```python
from build123d import *

# Parameters (mm, degrees)
SKETCH_1_R                = 2.15
EXTRUDE_1_DEPTH           = 4
SKETCH_2_R                = 16.75
SKETCH_2_R_2              = 1.65
CUT_EXTRUDE_1_DEPTH       = 10
CUT_EXTRUDE_2_DEPTH       = 10
FILLET_1_R                = 1.5
HOLE_WIZARD_1_D           = 3.4
HOLE_WIZARD_1_CSINK_D     = 6.6
HOLE_WIZARD_1_CSINK_ANGLE = 90


with BuildPart() as part:
    # 草图1 → 凸台-拉伸1 (new body)
    with BuildSketch(Plane.XY):
        with BuildLine():
            Line((-52, 30), (-52, 8.75))
            Line((-52, 8.75), (-52, -8.75))
            Line((-52, -8.75), (-52, -30))
            Line((-52, -30), (-47.54, -30))
            ThreePointArc((-47.54, -30), (-44.004466094, -31.464466094), (-42.54, -35))
            Line((-42.54, -35), (-42.54, -37.5))
            ThreePointArc((-42.54, -37.5), (-38.982425028, -42.287422066), (-33.372235985, -40.262198963))
            ThreePointArc((-33.372235985, -40.262198963), (-30.171244586, -38.118753147), (-26.396349665, -38.887436588))
            ThreePointArc((-26.396349665, -38.887436588), (0, -47), (26.396349665, -38.887436588))
            ThreePointArc((26.396349665, -38.887436588), (30.171244586, -38.118753147), (33.372235985, -40.262198963))
            ThreePointArc((33.372235985, -40.262198963), (38.674773042, -42.369526686), (42.499484755, -38.135225128))
            Line((42.499484755, -38.135225128), (46.619156699, -5.971116201))
            ThreePointArc((46.619156699, -5.971116201), (47, 0), (46.619156699, 5.971116201))
            Line((46.619156699, 5.971116201), (42.499484755, 38.135225128))
            ThreePointArc((42.499484755, 38.135225128), (38.674773042, 42.369526686), (33.372235985, 40.262198963))
            ThreePointArc((33.372235985, 40.262198963), (30.171244586, 38.118753147), (26.396349665, 38.887436588))
            ThreePointArc((26.396349665, 38.887436588), (0, 47), (-26.396349665, 38.887436588))
            ThreePointArc((-26.396349665, 38.887436588), (-30.171244586, 38.118753147), (-33.372235985, 40.262198963))
            ThreePointArc((-33.372235985, 40.262198963), (-38.982425028, 42.287422066), (-42.54, 37.5))
            Line((-42.54, 37.5), (-42.54, 35))
            ThreePointArc((-42.54, 35), (-44.004466094, 31.464466094), (-47.54, 30))
            Line((-47.54, 30), (-52, 30))
        make_face()
        with Locations((-37.54, -37.5)):
            Circle(SKETCH_1_R, mode=Mode.SUBTRACT)
        with Locations((37.54, -37.5)):
            Circle(SKETCH_1_R, mode=Mode.SUBTRACT)
        with Locations((-37.54, 37.5)):
            Circle(SKETCH_1_R, mode=Mode.SUBTRACT)
        with Locations((37.54, 37.5)):
            Circle(SKETCH_1_R, mode=Mode.SUBTRACT)
    extrude(amount=EXTRUDE_1_DEPTH)

    # 草图2 → 切除-拉伸1 (cut)
    with BuildSketch(Plane.XY.offset(4)):
        Circle(SKETCH_2_R)
        with Locations((0, 20)):
            Circle(SKETCH_2_R_2)
        with Locations((17.320508076, 10)):
            Circle(SKETCH_2_R_2)
        with Locations((17.320508076, -10)):
            Circle(SKETCH_2_R_2)
        with Locations((0, -20)):
            Circle(SKETCH_2_R_2)
        with Locations((-17.320508076, -10)):
            Circle(SKETCH_2_R_2)
        with Locations((-17.320508076, 10)):
            Circle(SKETCH_2_R_2)
    extrude(amount=-CUT_EXTRUDE_1_DEPTH, mode=Mode.SUBTRACT)

    # 草图3 → 切除-拉伸2 (cut)
    with BuildSketch(Plane.XY.offset(4)):
        with BuildLine():
            Line((-8.780014764, 22.872720449), (-10.751038486, 28.007412795))
            ThreePointArc((-10.751038486, 28.007412795), (-19.68177087, 22.641287407), (-26.238591214, 14.544288607))
            Line((-26.238591214, 14.544288607), (-21.428182825, 11.877835696))
            ThreePointArc((-21.428182825, 11.877835696), (-16.07344621, 18.490384715), (-8.780014764, 22.872720449))
        make_face()
        with BuildLine():
            Line((-1.282230928, 24.466423601), (-1.570078687, 29.958886043))
            ThreePointArc((-1.570078687, 29.958886043), (12.44079728, 27.298838126), (23.640322608, 18.46984426))
            Line((23.640322608, 18.46984426), (19.306263463, 15.083706145))
            ThreePointArc((19.306263463, 15.083706145), (10.159984445, 22.294051136), (-1.282230928, 24.466423601))
        make_face()
        with BuildLine():
            Line((23.022469209, 8.379493511), (28.190778624, 10.2606043))
            ThreePointArc((28.190778624, 10.2606043), (29.448815503, -5.724269861), (22.294344764, -20.073918191))
            Line((22.294344764, -20.073918191), (18.207048224, -16.393699856))
            ThreePointArc((18.207048224, -16.393699856), (24.049865994, -4.674820387), (23.022469209, 8.379493511))
        make_face()
        with BuildLine():
            Line((12.25, -21.217622393), (15, -25.980762114))
            ThreePointArc((15, -25.980762114), (-3.915785767, -29.743345841), (-21.213203436, -21.213203436))
            Line((-21.213203436, -21.213203436), (-17.324116139, -17.324116139))
            ThreePointArc((-17.324116139, -17.324116139), (-3.197891709, -24.290399104), (12.25, -21.217622393))
        make_face()
        with BuildLine():
            Line((-21.829659843, -11.122767244), (-26.730195726, -13.619714992))
            ThreePointArc((-26.730195726, -13.619714992), (-34.556729311, -2.576519476), (-47, 2.75))
            Line((-47, 2.75), (-47, 8.25))
            ThreePointArc((-47, 8.25), (-31.682987205, 2.113001428), (-21.829659843, -11.122767244))
        make_face()
        with BuildLine():
            Line((-12.722062209, 33.142105141), (-14.693085931, 38.276797486))
            ThreePointArc((-14.693085931, 38.276797486), (-26.898420189, 30.943092789), (-35.859407993, 19.87719443))
            Line((-35.859407993, 19.87719443), (-31.048999603, 17.210741519))
            ThreePointArc((-31.048999603, 17.210741519), (-23.290095529, 26.792190098), (-12.722062209, 33.142105141))
        make_face()
        with BuildLine():
            Line((-1.857926447, 35.451348484), (-2.145774206, 40.943810925))
            ThreePointArc((-2.145774206, 40.943810925), (17.002422949, 37.308412106), (32.308440898, 25.242120488))
            Line((32.308440898, 25.242120488), (27.974381753, 21.855982374))
            ThreePointArc((27.974381753, 21.855982374), (14.721610114, 32.303625116), (-1.857926447, 35.451348484))
        make_face()
        with BuildLine():
            Line((33.359088038, 12.141715088), (38.527397452, 14.022825876))
            ThreePointArc((38.527397452, 14.022825876), (40.246714521, -7.82316881), (30.468937845, -27.434354861))
            Line((30.468937845, -27.434354861), (26.381641304, -23.754136526))
            ThreePointArc((26.381641304, -23.754136526), (34.847765012, -6.773719336), (33.359088038, 12.141715088))
        make_face()
        with BuildLine():
            Line((17.75, -30.743901834), (20.5, -35.507041555))
            ThreePointArc((20.5, -35.507041555), (-5.351573881, -40.649239316), (-28.991378029, -28.991378029))
            Line((-28.991378029, -28.991378029), (-25.102290732, -25.102290732))
            ThreePointArc((-25.102290732, -25.102290732), (-4.633679824, -35.196292579), (17.75, -30.743901834))
        make_face()
        with BuildLine():
            Line((-31.630731609, -16.116662741), (-36.531267492, -18.613610489))
            ThreePointArc((-36.531267492, -18.613610489), (-40.304213522, -11.955561283), (-47, -8.25))
            Line((-47, -8.25), (-47, -2.75))
            ThreePointArc((-47, -2.75), (-37.430471416, -7.266040379), (-31.630731609, -16.116662741))
        make_face()
    extrude(amount=-CUT_EXTRUDE_2_DEPTH, mode=Mode.SUBTRACT)

    # 圆角1
    fillet_1_edges = [part.edges().sort_by_distance(p)[0] for p in [
        (-47, 8.25, 2),
        (-21.829659843, -11.122767244, 2),
        (-26.730195726, -13.619714992, 2),
        (-47, 2.75, 2),
        (-35.859407993, 19.87719443, 2),
        (-14.693085931, 38.276797486, 2),
        (-12.722062209, 33.142105141, 2),
        (-31.048999603, 17.210741519, 2),
        (-17.324116139, -17.324116139, 2),
        (12.25, -21.217622393, 2),
        (15, -25.980762114, 2),
        (-21.213203436, -21.213203436, 2),
        (20.5, -35.507041555, 2),
        (-28.991378029, -28.991378029, 2),
        (-25.102290732, -25.102290732, 2),
        (17.75, -30.743901834, 2),
        (-1.570078687, 29.958886043, 2),
        (23.640322608, 18.46984426, 2),
        (19.306263463, 15.083706145, 2),
        (-1.282230928, 24.466423601, 2),
        (26.381641304, -23.754136526, 2),
        (33.359088038, 12.141715088, 2),
        (38.527397452, 14.022825876, 2),
        (30.468937845, -27.434354861, 2),
        (27.974381753, 21.855982374, 2),
        (-1.857926447, 35.451348484, 2),
        (-2.145774206, 40.943810925, 2),
        (32.308440898, 25.242120488, 2),
        (-8.780014764, 22.872720449, 2),
        (-21.428182825, 11.877835696, 2),
        (-26.238591214, 14.544288607, 2),
        (-10.751038486, 28.007412795, 2),
        (-36.531267492, -18.613610489, 2),
        (-47, -8.25, 2),
        (-47, -2.75, 2),
        (-31.630731609, -16.116662741, 2),
        (28.190778624, 10.2606043, 2),
        (22.294344764, -20.073918191, 2),
        (18.207048224, -16.393699856, 2),
        (23.022469209, 8.379493511, 2),
    ]]
    fillet(fillet_1_edges, radius=FILLET_1_R)

    # 打孔尺寸(%根据十字)槽半沉头木螺钉的类型1 (through all)
    with Locations(Plane(origin=(-17.320508076, 10, 4), x_dir=(1, 0, 0), z_dir=(0, 0, 1))):
        with Locations((0, 0), (17.320508076, 10), (34.641016152, 0), (34.641016152, -20), (17.320508076, -30), (0, -20)):
            CounterSinkHole(HOLE_WIZARD_1_D / 2, HOLE_WIZARD_1_CSINK_D / 2, counter_sink_angle=HOLE_WIZARD_1_CSINK_ANGLE)


solid = part.part
```
Can you work these out from the model? Positions are in its coordinate system, mm. A direction names the side the tool comes from. Round coordinates to 2 decimals unless told otherwise and drop trailing zeros. Loops run counter-clockwise (first coordinate to the right, second up) from the corner with the lowest first, then second, coordinate; pieces in that order, holes last.
Item 1: Suppose I cut it at C-C, the plane z = 1.5. State how many separate pieces and enclosed holes the cut face has, then the cut area to 3 significant figures.
Item 2: Suppose I cut it at B-B, the plane y = 0. Write out the boundary of the cut face in (x, z), then the cut area to 3 significant figures.
Item 3: If we mould it in two halves opening along Y, with no side actions, what happens to faces 3 (the cylindrical face through (-36, 39, 2)), 4 (the cylindrical face through (34.8, -7.02, 2.03)), 5 (the cylindrical face through (-44.04, -31.43, 1.97))? For each: +Y half, -Y half, draft (parallel to the pull), parting line (faces both ways), or undercut.
Item 4: Will these pins go through, and if not, where does the flat tip stop? pin 1 Ø1.2 at (x, z) = (-49.5, 2.5) entering from -Y; pin 2 Ø1.2 at (x, z) = (-49, 2.5) entering from +Y; pin 3 Ø1 at (y, z) = (11, 2) entering from +X.
Item 5: Suppose I cut it at A-A, the plane x = 6. Write out the boundary of the cut face in (y, z), then the cut area to 3 significant figures.
Item 6: Which directions (+Z, -Z, +X, -X, +Y, -Y) give clear straight access to the entire face, cutting with the end or side of a thin tool? Please do faces 1 (the cylindrical face through (-5.001, -40.694, 2.028)), 2 (the flat face through (-50, -30, 2)).
Item 7: Please list where these lines run through material, in increasing order: L1, parallel to X at y = 0, z = 1.5; L2, parallel to X at y = 10, z = 1.35; L3, parallel to Y at x = 11, z = 3.7.
Reported:
1. separate pieces: 1
1. enclosed holes: 21
1. area: 5,350 mm2
2. outline: (-52, 0) - (-38.44, 0) - (-38.44, 4) - (-52, 4) - close; (-29.22, 0) - (-16.75, 0) - (-16.75, 4) - (-29.22, 4) - close; (16.75, 0) - (24.5, 0) - (24.5, 4) - (16.75, 4) - close; (30, 0) - (35.5, 0) - (35.5, 4) - (30, 4) - close; (41, 0) - (47, 0) - (47, 4) - (41, 4) - close
2. area: 181 mm2
3. face 3: undercut
3. face 4: undercut
3. face 5: -Y half
4. pin 1: stops at y = -30
4. pin 2: stops at y = 30
4. pin 3: stops at x = 46.04
5. outline: (-46.62, 0) - (-40.56, 0) - (-40.56, 4) - (-46.62, 4) - close; (-34.99, 0) - (-29.39, 0) - (-29.39, 4) - (-34.99, 4) - close; (-23.75, 0) - (-15.64, 0) - (-15.64, 4) - (-23.75, 4) - close; (15.64, 0) - (23.75, 0) - (23.75, 4) - (15.64, 4) - close; (29.39, 0) - (34.99, 0) - (34.99, 4) - (29.39, 4) - close; (40.56, 0) - (46.62, 0) - (46.62, 4) - (40.56, 4) - close
5. area: 158 mm2
6. face 1: +Z, -Z
6. face 2: +Z, -Z, -X, -Y
7. L1: x = -52 to -38.44, -29.22 to -16.75, 16.75 to 24.5, 30 to 35.5, 41 to 47
7. L2: x = -52 to -19.02, -15.62 to -13.44, 13.44 to 15.62, 19.02 to 34.06, 39.76 to 46.1
7. L3: y = -45.69 to -39.5, -33.75 to -27.91, -21.89 to -12.63, 12.63 to 21.89, 27.91 to 33.75, 39.5 to 45.69
